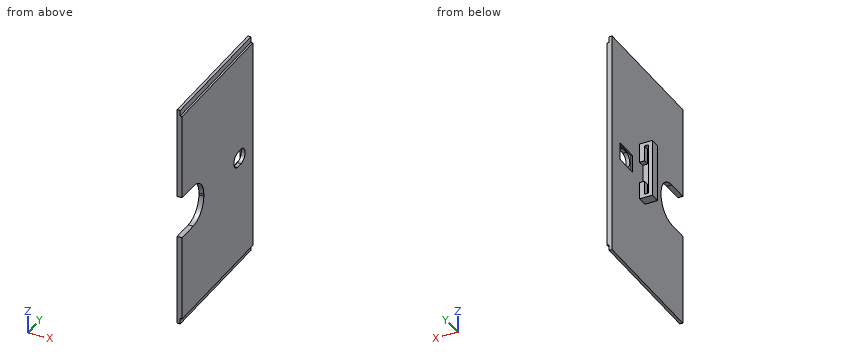
```python
from build123d import *

# Parameters (mm, degrees)
SKETCH_1_W           = 120
SKETCH_1_H           = 68
EXTRUDE_1_DEPTH      = 3
CUT_EXTRUDE_1_DEPTH  = 91.735880444
CUT_EXTRUDE_7_DEPTH  = 2.5
CUT_EXTRUDE_10_DEPTH = 2.5
SKETCH_17_W          = 9
SKETCH_17_H          = 12
CUT_EXTRUDE_11_DEPTH = 0.65
EXTRUDE_2_DEPTH      = 8
SKETCH_19_W          = 1.564505321
SKETCH_19_H          = 29.5
CUT_EXTRUDE_12_DEPTH = 8
EXTRUDE_3_DEPTH      = 3


with BuildPart() as part:
    # 스케치1 → 보스-돌출1 (new body)
    with BuildSketch(Plane(origin=(0, 0, 0), x_dir=(0, 0, -1), z_dir=(1, 0, 0))):
        Rectangle(SKETCH_1_W, SKETCH_1_H)
    extrude(amount=EXTRUDE_1_DEPTH)

    # 스케치2 → 컷-돌출1 (cut, through all)
    with BuildSketch(Plane(origin=(0, 34, 0), x_dir=(1, 0, 0), z_dir=(0, 1, 0))):
        Polygon((0.5, -60), (0.5, -57.5), (0.5, 0), (0, 0), (0, -60), align=None)
        Polygon((2, -57.5), (0.5, -57.5), (0.5, -60), (3, -60), (3, -54.5), (2, -54.5), align=None)
        Polygon((0.5, 60), (0.5, 57.5), (2, 57.5), (2, 54.5), (3, 54.5), (3, 60), align=None)
        Polygon((0, 0), (0.5, 0), (0.5, 57.5), (0.5, 60), (0, 60), align=None)
    extrude(amount=-CUT_EXTRUDE_1_DEPTH, mode=Mode.SUBTRACT)

    # 스케치7 → 컷-돌출7 (cut)
    with BuildSketch(Plane(origin=(3, 0, 0), x_dir=(0, 0, -1), z_dir=(1, 0, 0))):
        with BuildLine():
            Line((0.5, -13.133811576), (-0.5, -13.133811576))
            ThreePointArc((-0.5, -13.133811576), (-7.747844507, -16.135967068), (-10.75, -23.383811576))
            Line((-10.75, -23.383811576), (-10.75, -34))
            Line((-10.75, -34), (10.75, -34))
            Line((10.75, -34), (10.75, -23.383811576))
            ThreePointArc((10.75, -23.383811576), (7.747844507, -16.135967068), (0.5, -13.133811576))
        make_face()
    extrude(amount=-CUT_EXTRUDE_7_DEPTH, mode=Mode.SUBTRACT)

    # 스케치16 → 컷-돌출10 (cut)
    with BuildSketch(Plane(origin=(3, 0, 0), x_dir=(0, 0, -1), z_dir=(1, 0, 0))):
        with BuildLine():
            Line((-3.875, 22.666188424), (-3.82691794, 19.057645835))
            ThreePointArc((-3.82691794, 19.057645835), (0, 15.791188424), (3.82691794, 19.057645835))
            Line((3.82691794, 19.057645835), (3.875, 22.666188424))
            ThreePointArc((3.875, 22.666188424), (0, 26.541188424), (-3.875, 22.666188424))
        make_face()
    extrude(amount=-CUT_EXTRUDE_10_DEPTH, mode=Mode.SUBTRACT)

    # 스케치17 → 컷-돌출11 (cut)
    with BuildSketch(Plane.ZY.offset(-0.5)):
        with Locations((0, 20.55)):
            Rectangle(SKETCH_17_W, SKETCH_17_H)
    extrude(amount=-CUT_EXTRUDE_11_DEPTH, mode=Mode.SUBTRACT)

    # 스케치18 → 보스-돌출2 (add)
    with BuildSketch(Plane.ZY.offset(-0.5)):
        Polygon((-12.5, 4.5), (-14.75, 4.5), (-14.75, 2.5), (0, 2.5), (0, 4.5), align=None)
        Polygon((12.5, 4.5), (0, 4.5), (0, 2.5), (14.75, 2.5), (14.75, 4.5), align=None)
    extrude(amount=EXTRUDE_2_DEPTH)

    # 스케치19 → 컷-돌출12 (cut)
    with BuildSketch(Plane(origin=(0, 4.5, 0), x_dir=(1, 0, 0), z_dir=(0, 1, 0))):
        with Locations((-6.71774734, 0)):
            Rectangle(SKETCH_19_W, SKETCH_19_H)
    extrude(amount=-CUT_EXTRUDE_12_DEPTH, mode=Mode.SUBTRACT)

    # 스케치19<3> → 보스-돌출3 (add)
    with BuildSketch(Plane(origin=(0, 4.5, 0), x_dir=(1, 0, 0), z_dir=(0, 1, 0))):
        Polygon((0.5, 6), (0.5, 14.75), (-5.935494679, 14.75), (-5.935494679, -14.75), (0.5, -14.75), (0.5, -5), (-1.935494679, -5), (-1.935494679, -13), (-3.935494679, -13), (-3.935494679, 13), (-1.935494679, 13), (-1.935494679, 6), align=None)
    extrude(amount=EXTRUDE_3_DEPTH)


solid = part.part
```
Part model, mm, in its own coordinate system. Round coordinates to 2 decimals unless told otherwise and drop trailing zeros. Order: outer loops, then holes, each group sorted by start corner. A loop starts at its lowest first (then second) coordinate and runs counter-clockwise, first axis right, second up. Notation, with made-up numbers: M 22,57.25 L 78,57.25 A26 ccw 78,84.25 Z; hole C 1.5,6.25 d2. An arc over 180 degrees is marked long. Put each result on its own line as item: value. Start each with the question number.
1. Slice it at A-A on y = -17. List the corners of the cut face in (x, z).
2. Drop flat-ended pins along their axis: pin 1 (2 mm diameter, centred on x = -1, z = 5.5, fed in from +Y); pin 2 (1 mm diameter, centred on x = -2.5, y = 6, fed in from +Z); pin 3 (5 mm diameter, centred on x = -3, z = -9, fed in from -Y). Give the stop position or say it passes through.
3. Drill centre lines: probe 1 along X at (y, z) = (30.5, -46); probe 2 along Z at (x, y) = (0.75, -14); probe 3 along Y at (x, z) = (-4.5, -12.5). Where is each one in solid material? Low to high. Write a range as [from, to].
4. Slice it at B-B on y = 9.5. List the corners of the cut face in (x, z).
5. Slice it at C-C on z = 18.5. List the corners of the cut face in (x, y), then the cut area to 3 significant figures.
Findings:
1. outline: M 0.5,-57.5 L 2,-57.5 L 2,-54.5 L 3,-54.5 L 3,-8.52 L 0.5,-8.52 Z; M 0.5,8.52 L 3,8.52 L 3,54.5 L 2,54.5 L 2,57.5 L 0.5,57.5 Z
2. pin 1: y = 7.5
2. pin 2: z = 14.75
2. pin 3: y = 2.5
3. probe 1: [0.5, 3]
3. probe 2: [-57.5, -4.62], [4.62, 57.5]
3. probe 3: [2.5, 7.5]
4. outline: M 0.5,-57.5 L 2,-57.5 L 2,-54.5 L 3,-54.5 L 3,54.5 L 2,54.5 L 2,57.5 L 0.5,57.5 Z
5. outline: M 0.5,-34 L 3,-34 L 3,34 L 0.5,34 Z
5. area: 170 mm2
